Input: part model. Units: mm. Frame: model coordinates. Coordinates: 2 decimals unless noted, no trailing zeros. Loops run counter-clockwise (first coordinate to the right, second up) from the corner with the lowest first, then second, coordinate; pieces in that order, holes last. Notation, with made-up numbers: M 75,-14.75 L 98,-14.75 A3 ccw 98,-9.75 Z; hole C 4,53.5 d2. An arc over 180 degrees is marked long. Use a Markdown table: item, result. Add a question column.
1. Section A-A on x = -31. Output: boundary loops of the cut face in (y, z).
2. Pin query (flat end, axial travel): pin 1 (5.5 mm diameter, centred on y = -137, z = 169, fed in from +X). Return the tip coordinate at first contact, or that it passes through.
3. Section B-B on z = 207.5. Output: boundary loops of the cut face in (x, y).
4. Line query: L1, parallel to Y at x = -26.75, z = 73; L2, parallel to X at y = -135, z = 194. Output: solid intervals per line, ascending. Write a range as [from, to].
5. Section C-C on y = -136.5. Output: boundary loops of the cut face in (x, z).
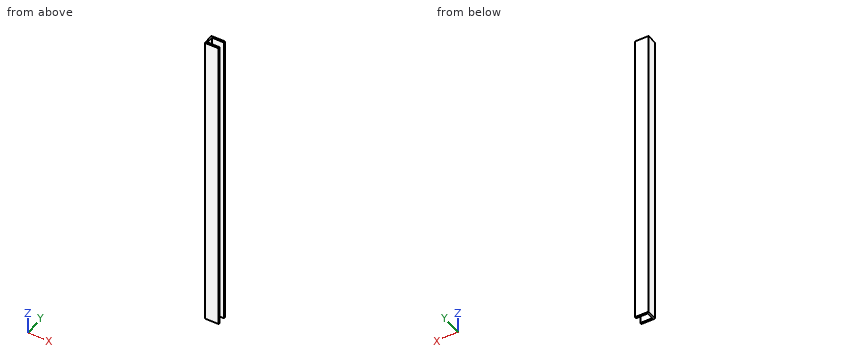
Autodesk Inventor part; units mm, degrees
ref_plane "YZ Plane" through (0, 0, 0) normal (1, 0, 0) x (0, 1, 0)
ref_plane "XZ Plane" through (0, 0, 0) normal (0, 1, 0) x (-1, 0, 0)
ref_plane "XY Plane" through (0, 0, 0) normal (0, 0, 1) x (1, 0, 0)
ref_plane "Work Plane1" through (23.8016, -120.6016, 287.3377) normal (0, 0, 1) x (1, 0, 0)
sketch "Sketch1" plane through (23.8016, -120.6016, 287.3377) normal (0, 0, 1) x (1, 0, 0)
  line L0 (-60.325, -11.1235) -> (-60.325, -21.1235)
  line L1 (-60.325, -21.1235) -> (-47.325, -21.1235)
  line L2 (-47.325, -21.1235) -> (-47.325, -19.5235)
  line L3 (-47.325, -19.5235) -> (-58.725, -19.5235)
  line L4 (-58.725, -19.5235) -> (-58.725, -12.7235)
  line L5 (-58.725, -12.7235) -> (-47.3247, -12.7235)
  line L6 (-47.3247, -12.7235) -> (-47.3247, -11.1235)
  line L7 (-47.3247, -11.1235) -> (-60.325, -11.1235)
  point P0 (-23.8016, 120.6016)
  dimension "d0" = 10
  dimension "d1" = 13
  dimension "d2" = 1.6
  dimension "d3" = 1.6
  dimension "d4" = 1.6
extrude "Extrusion1" add sketch "Sketch1" against normal blind 286.324
properties part number "Z-table Rail"
Answers below:
| question | item | result |
|---|---|---|
| 1 | outline | M -141.73,1.01 L -140.13,1.01 L -140.13,287.34 L -141.73,287.34 Z; M -133.33,1.01 L -131.73,1.01 L -131.73,287.34 L -133.33,287.34 Z |
| 2 | pin 1 | stops at x = -34.92 |
| 3 | outline | M -36.52,-141.73 L -23.52,-141.73 L -23.52,-140.13 L -34.92,-140.13 L -34.92,-133.33 L -23.52,-133.33 L -23.52,-131.73 L -36.52,-131.73 Z |
| 4 | L1 | y = [-141.73, -140.13], [-133.33, -131.73] |
| 4 | L2 | x = [-36.52, -34.92] |
| 5 | outline | M -36.52,1.01 L -34.92,1.01 L -34.92,287.34 L -36.52,287.34 Z |
